```python
from build123d import *

# Parameters (mm, degrees)
F0_W     = 101.6
F0_H     = 88.9
F1_DEPTH = 3.175
F2_W     = 3.175
F2_H     = 88.9
F3_DEPTH = 101.6
F4_W     = 3.175
F4_H     = 88.9
F5_DEPTH = 98.425
F6_R     = 3.175
F7_R     = 1.905
F8_DEPTH = 104.776


with BuildPart() as f1:
    # F0 (on Front) → F1 (new body)
    with BuildSketch(Plane.XZ):
        with Locations((50.8, 44.45)):
            Rectangle(F0_W, F0_H)
    extrude(amount=F1_DEPTH)

    # F2 (on face) → F3 (join)
    with BuildSketch(Plane.XZ.offset(3.175)):
        with Locations((1.5875, 44.45)):
            Rectangle(F2_W, F2_H)
    extrude(amount=F3_DEPTH)

    # F4 (on face) → F5 (join, through all)
    with BuildSketch(Plane.YZ.offset(3.175)):
        with Locations((-103.1875, 44.45)):
            Rectangle(F4_W, F4_H)
    extrude(amount=F5_DEPTH)

    # F6
    f6_edges = [f1.edges().sort_by_distance(p)[0] for p in [
        (0, 0, 44.45),
        (0, -104.775, 44.45),
    ]]
    fillet(f6_edges, radius=F6_R)

    # F7 (on face) → F8 (cut, through all)
    with BuildSketch(Plane.XZ.offset(104.775)):
        with Locations((38.1, 83.312)):
            Circle(F7_R)
        with Locations((50.8, 83.312)):
            Circle(F7_R)
        with Locations((63.5, 83.312)):
            Circle(F7_R)
    extrude(amount=-F8_DEPTH, mode=Mode.SUBTRACT)


solid = f1.part
```
Work out the finished part from the listing and answer in its coordinate system (mm). A direction names the side the tool comes from. Give positions to 0.01 mm unless a question says otherwise; leave off trailing zeros. Write each loop counter-clockwise with the first axis right and the second up, starting at its lowest first coordinate (ties: lowest second). Pieces come first, ordered by that corner, then holes. Notation, with made-up numbers: (78, 26.5) - (88, 26.5) arc R25 cw to (88, 58.5) - close; hole circle Ø6 at (-39, -7.75). An arc over 180 degrees is marked (long way). Use one line per item in the form item = value.
1. For faces 5 (the face through (52, -3.175, 45)), 6 (the face through (52, -104.775, 44)), determine the directions among +Z, -Z, +X, -X, +Y, -Y from which every point of the face is accessible in a straight line to the end or side of a thin tool.
Filled in:
face_5 = +Z, -Z, +X
face_6 = +Z, -Z, +X, -X, -Y
2. Determine the mould class of faces 1 (the face through (3.175, -52, 44)), 2 (the face through (0.955, -103.87, 45.072)), 3 (the face through (52.62, -103.21, 83.88)), 4 (the face through (39.92, -103.21, 83.88)) for opening direction X: released by +X, released by -X, zero draft, split by the parting line, or undercut.
Filled in:
face_1 = released by +X
face_2 = released by -X
face_3 = undercut
face_4 = undercut
3. A cutting plane is placed at C-C (y = -20). Write down the section's boundary in (x, z) (3 decimals).
Filled in:
outline = (0, 0) - (3.175, 0) - (3.175, 88.9) - (0, 88.9) - close
4. Each of these flat-tipped pins is pushed along its axis until it touches: pin 1 Ø6 at (y, z) = (-65.5, 53.5) entering from +X (3 decimals); pin 2 Ø6 at (x, z) = (38.1, 83.312) entering from +Y. Where does it stop, or does it pass through?
Filled in:
pin_1 = 3.175
pin_2 = 0
5. A cutting plane is placed at B-B (z = 33). Write down the section's boundary in (x, y) (3 decimals).
Filled in:
outline = (0, -101.6) arc R3.175 ccw to (3.175, -104.775) - (101.6, -104.775) - (101.6, -101.6) - (3.175, -101.6) - (3.175, -3.175) - (101.6, -3.175) - (101.6, 0) - (3.175, 0) arc R3.175 ccw to (0, -3.175) - close
6. Consider L1, parallel to Y at x = 67.5, z = 56 (3 decimals); L2, parallel to Z at x = 38.1, y = -2.5; L3, parallel to X at y = -101, z = 62 (3 decimals). Determine where each line is inside the solid, lowest interval first.
Filled in:
L1 = -104.775 to -101.6, -3.175 to 0
L2 = 0 to 81.41, 85.22 to 88.9
L3 = 0 to 3.175
7. A cutting plane is placed at A-A (x = 44). Write down the section's boundary in (y, z) (3 decimals).
Filled in:
outline = (-104.775, 0) - (-101.6, 0) - (-101.6, 88.9) - (-104.775, 88.9) - close; (-3.175, 0) - (0, 0) - (0, 88.9) - (-3.175, 88.9) - close
